The listing builds one solid part. Answer for the finished solid, in the listing's coordinates (mm). A direction names the side the tool comes from. Give positions to 0.01 mm unless a question says otherwise; leave off trailing zeros. Write each loop counter-clockwise with the first axis right and the second up, starting at its lowest first coordinate (ties: lowest second). Pieces come first, ordered by that corner, then holes. Notation, with made-up numbers: M 51,-11.75 L 76,-11.75 A24 cw 76,6.25 Z; hole C 50,60 d7. An arc over 180 degrees is marked long. Answer as a JSON object with one key per item and string values.
```python
from build123d import *

# Parameters (mm, degrees)
SKETCH1_R                 = 3
BOSS_EXTRUDE3_DEPTH       = 4
BOSS_EXTRUDE3_2_DEPTH     = 4
BOSS_EXTRUDE3_3_DEPTH     = 4
BOSS_EXTRUDE3_4_DEPTH     = 4
SKETCH1_6_R               = 11
SKETCH1_6_R_2             = 3
SKETCH1_6_R_3             = 7.5
BOSS_EXTRUDE9_DEPTH       = 1
SKETCH5_R                 = 2
CUT_EXTRUDE5_DEPTH        = 2
SKETCH9_R                 = 9.5
BOSS_EXTRUDE17_DEPTH      = 2
BOSS_EXTRUDE17_DEPTH_BACK = 0.0001
CUT_EXTRUDE11_START       = -0.5
SKETCH24_R                = 9
CUT_EXTRUDE11_DEPTH       = 1
FILLET10_R                = 1
SKETCH11_R                = 1
CUT_EXTRUDE13_DEPTH       = 2.5
CUT_EXTRUDE14_START       = -1
SKETCH26_R                = 1
CUT_EXTRUDE14_DEPTH       = 5.5
FILLET11_R                = 1


with BuildPart() as part:
    # Sketch1 → Boss-Extrude3 (new body)
    with BuildSketch(Plane.XY):
        with Locations((0, 7.5)):
            Circle(SKETCH1_R)
    extrude(amount=BOSS_EXTRUDE3_DEPTH)



with BuildPart() as body_2:
    # Sketch1 → Boss-Extrude3 2 (new body)
    with BuildSketch(Plane.XY):
        with Locations((0, -7.5)):
            Circle(SKETCH1_R)
    extrude(amount=BOSS_EXTRUDE3_2_DEPTH)


with BuildPart() as body_3:
    # Sketch1 → Boss-Extrude3 3 (new body)
    with BuildSketch(Plane.XY):
        with Locations((-7.5, 0)):
            Circle(SKETCH1_R)
    extrude(amount=BOSS_EXTRUDE3_3_DEPTH)


with BuildPart() as body_4:
    # Sketch1 → Boss-Extrude3 4 (new body)
    with BuildSketch(Plane.XY):
        with Locations((7.5, 0)):
            Circle(SKETCH1_R)
    extrude(amount=BOSS_EXTRUDE3_4_DEPTH)


with BuildPart() as part_1:
    add(part.part)

    add(body_2.part)  # Boss-Extrude9 merges body 2

    add(body_3.part)  # Boss-Extrude9 merges body 3

    add(body_4.part)  # Boss-Extrude9 merges body 4
    # Sketch1_6 → Boss-Extrude9 (add)
    with BuildSketch(Plane.XY):
        Circle(SKETCH1_6_R)
        with Locations((7.5, 0)):
            Circle(SKETCH1_6_R_2, mode=Mode.SUBTRACT)
        Circle(SKETCH1_6_R_3, mode=Mode.SUBTRACT)
        with Locations((0, -7.5)):
            Circle(SKETCH1_6_R_2, mode=Mode.SUBTRACT)
        with Locations((-7.5, 0)):
            Circle(SKETCH1_6_R_2, mode=Mode.SUBTRACT)
        with Locations((0, 7.5)):
            Circle(SKETCH1_6_R_2, mode=Mode.SUBTRACT)
        with Locations((7.5, 0)):
            Circle(SKETCH1_6_R_2)
        Circle(SKETCH1_6_R_3)
        with Locations((0, 7.5)):
            Circle(SKETCH1_6_R_2)
        with Locations((-7.5, 0)):
            Circle(SKETCH1_6_R_2)
        with Locations((0, -7.5)):
            Circle(SKETCH1_6_R_2)
    extrude(amount=BOSS_EXTRUDE9_DEPTH)

    # Sketch5 → Cut-Extrude5 (cut)
    with BuildSketch(Plane.XY.offset(4)):
        with Locations((0, 7.5)):
            Circle(SKETCH5_R)
        with Locations((7.5, 0)):
            Circle(SKETCH5_R)
        with Locations((0, -7.5)):
            Circle(SKETCH5_R)
        with Locations((-7.5, 0)):
            Circle(SKETCH5_R)
    extrude(amount=-CUT_EXTRUDE5_DEPTH, mode=Mode.SUBTRACT)

    # Sketch9 → Boss-Extrude17 (add, two sides)
    with BuildSketch(Plane(origin=(0, 0, 0), x_dir=(-1, 0, 0), z_dir=(0, 0, -1))) as boss_extrude17_sk:
        Circle(SKETCH9_R)
    extrude(amount=BOSS_EXTRUDE17_DEPTH)
    extrude(boss_extrude17_sk.sketch, amount=-BOSS_EXTRUDE17_DEPTH_BACK)

    # Sketch24 → Cut-Extrude11 (cut)
    with BuildSketch(Plane(origin=(0, 0, -2), x_dir=(-1, 0, 0), z_dir=(0, 0, -1)).offset(CUT_EXTRUDE11_START)):
        Circle(SKETCH24_R)
    extrude(amount=-CUT_EXTRUDE11_DEPTH, mode=Mode.SUBTRACT)

    # Fillet10
    fillet10_edges = [part_1.edges().sort_by_distance(p)[0] for p in [
        (9.5, 0, 0),
    ]]
    fillet(fillet10_edges, radius=FILLET10_R)

    # Sketch11 → Cut-Extrude13 (cut)
    with BuildSketch(Plane.XY.offset(2)):
        with Locations((0, 7.5)):
            Circle(SKETCH11_R)
        with Locations((-7.5, 0)):
            Circle(SKETCH11_R)
        with Locations((0, -7.5)):
            Circle(SKETCH11_R)
        with Locations((7.5, 0)):
            Circle(SKETCH11_R)
    extrude(amount=-CUT_EXTRUDE13_DEPTH, mode=Mode.SUBTRACT)

    # Sketch29 → Revolve3 (revolve)
    with BuildSketch(Plane(origin=(0, 0, 0), x_dir=(0, 0, -1), z_dir=(1, 0, 0))):
        Polygon((2, 0), (2, 2), (5.5, 1.5), (5.5, 0), align=None)
    revolve(axis=Axis((0, 0, -2), (0, 0, -1)))

    # Sketch26 → Cut-Extrude14 (cut, through all)
    with BuildSketch(Plane(origin=(0, 0, -2), x_dir=(-1, 0, 0), z_dir=(0, 0, -1)).offset(CUT_EXTRUDE14_START)):
        Circle(SKETCH26_R)
    extrude(amount=CUT_EXTRUDE14_DEPTH, mode=Mode.SUBTRACT)

    # Fillet11
    fillet11_edges = [part_1.edges().sort_by_distance(p)[0] for p in [
        (0, -2, -2),
    ]]
    fillet(fillet11_edges, radius=FILLET11_R)


solid = part_1.part
```
1. The mould has two halves that part along Y. Classify faces 5 (the cylindrical face through (-2.38, -10.74, 0.49)), 6 (the flat face through (4, -10, 0)), 7 (the cylindrical face through (6.7, -0.6, 0.8)): released by +Y, released by -Y, zero draft, split by the parting line, or undercut.
Verdict:
{"face 5": "split by the parting line", "face 6": "zero draft", "face 7": "undercut"}
2. Consider line 1 along Y through (x, z) = (0, 3.3); line 2 along X through (y, z) = (0.75, 0.25); line 3 along Z through (x, y) = (-4.5, -5.5). Determine where each line is inside the solid, lowest interval first.
Verdict:
{"line 1": "y = -10.5 to -9.5, -5.5 to -4.5, 4.5 to 5.5, 9.5 to 10.5", "line 2": "x = -10.97 to -8.16, -6.84 to 6.84, 8.16 to 10.97", "line 3": "z = -2 to -1.5, -0.5 to 1"}
3. A cutting plane is placed at A-A, the plane z = 3.25. Give the vertices of the cut face in (x, y), plus the area to 3 significant figures.
Verdict:
{"outline": "C -7.5,0 d6; C 0,-7.5 d6; C 0,7.5 d6; C 7.5,0 d6; hole C -7.5,0 d4; hole C 0,-7.5 d4; hole C 0,7.5 d4; hole C 7.5,0 d4", "area": "62.8 mm2"}
4. A cutting plane is placed at B-B, the plane x = 0. Count the separate pieces of the cut face and the enclosed holes in it, plus the area to 3 significant figures.
Verdict:
{"separate pieces": "3", "enclosed holes": "0", "area": "57.0 mm2"}
5. For faces 1 (the flat face through (5, 0, 4)), 2 (the flat face through (2.2, 2.2, -2)), 3 (the flat face through (0, -2, -1.5)), 4 (the cylindrical face through (-0.26, 9.483, 3.014)), determine the directions among +Z, -Z, +X, -X, +Y, -Y from which every point of the face is accessible in a straight line to the end or side of a thin tool.
Verdict:
{"face 1": "+Z, +X, -X, +Y, -Y", "face 2": "-Z", "face 3": "none", "face 4": "+Z"}
6. Flat-ended cylindrical pins translate along their axes: pin 1 (4.5 mm diameter, centred on x = -1, y = -8, fed in from +Z); pin 2 (1.2 mm diameter, centred on x = -8.5, y = 0.5, fed in from +Z); pin 3 (1.8 mm diameter, centred on x = 0, y = 0, fed in from -Z); pin 4 (2.5 mm diameter, centred on x = 0, y = 7.5, fed in from -Z). Find the tip coordinate at first contact, or state that the pin passes through.
Verdict:
{"pin 1": "stops at z = 4", "pin 2": "stops at z = 2", "pin 3": "stops at z = -0.5", "pin 4": "stops at z = -2"}
